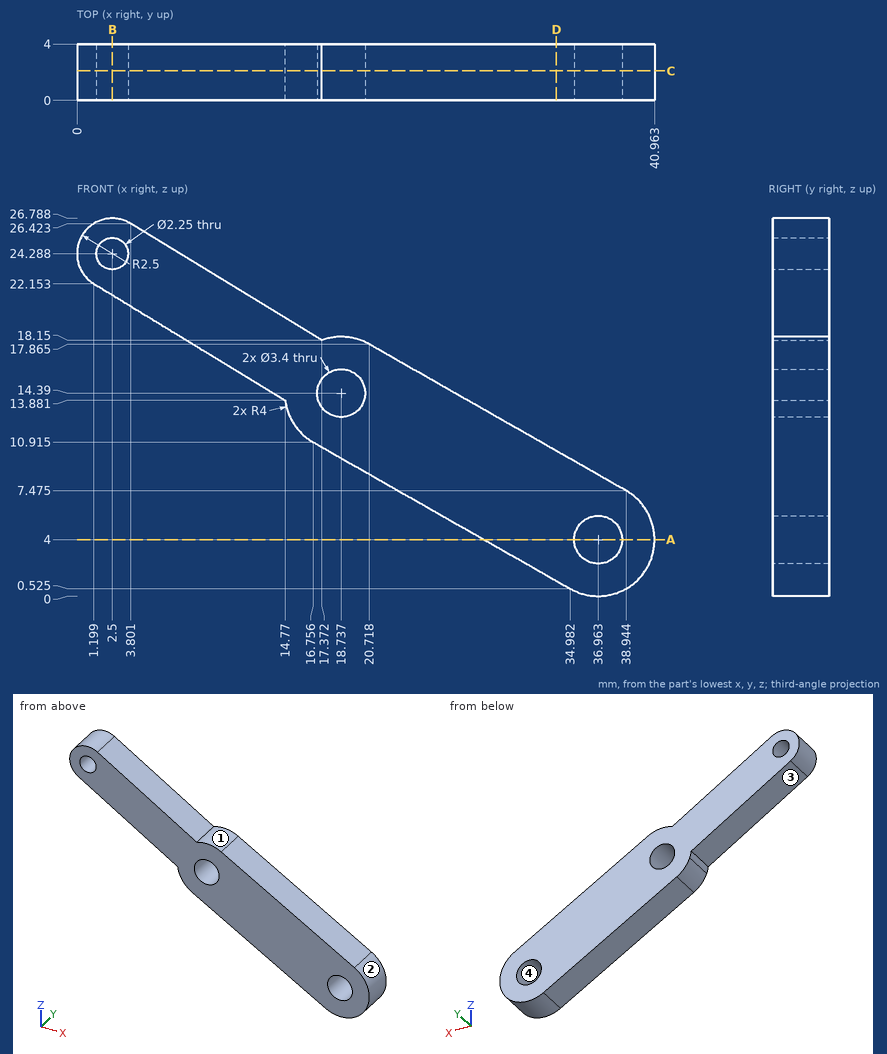
Here's the drawing with two shaded views (mm, measured from the low corner). I have some questions. Round coordinates to 2 decimals unless told otherwise and drop trailing zeros. Write each loop counter-clockwise with the first axis right and the second up, starting at its lowest first coordinate (ties: lowest second). Pieces come first, ordered by that corner, then holes. Notation, with made-up numbers: M 41,-18.5 L 46,-18.5 A23 cw 46,1.5 Z; hole C 56.5,-1.75 d4. An arc over 180 degrees is marked long. Use CSV: the item, a comma, the result in double quotes.
(1) Imagine slicing it at D-D (x = 34). Write out the boundary of the cut face in (y, z) (1 decimal).
Check values:
outline,"M 0,1.1 L 4,1.1 L 4,10.3 L 0,10.3 Z"
(2) We'd pull the mould along X, two halves only. Please class the marked faces 1, 2, 3 and 4: +X half, -X half, draft (parallel to the pull), parting line (faces both ways), or undercut.
Check values:
face 1,"undercut"
face 2,"parting line"
face 3,"-X half"
face 4,"undercut"
(3) Imagine slicing it at C-C (y = 2.1). Count the separate pieces of the cut face and the enclosed holes in it, plus the area to 3 significant figures.
Check values:
separate pieces,"1"
enclosed holes,"3"
area,"282 mm^2"
(4) I need wall thicknesses on line 1 along X through (y, z) = (1.95, 14) (1 decimal); line 2 along X through (y, z) = (2.15, 24.75) (1 decimal); line 3 along X through (y, z) = (2, 16.5) (1 decimal). Which ranges of each line are inside material? Lowest first, please.
Check values:
line 1,"14.6 to 17.1, 20.4 to 27.5"
line 2,"0 to 1.5, 3.5 to 6.5"
line 3,"10.5 to 23.1"
(5) Imagine slicing it at B-B (x = 2.5). Write out the boundary of the cut face in (y, z), plus the area to 3 significant figures.
Check values:
outline,"M 0,21.36 L 4,21.36 L 4,23.16 L 0,23.16 Z; M 0,25.41 L 4,25.41 L 4,26.79 L 0,26.79 Z"
area,"12.7 mm^2"
(6) Imagine slicing it at A-A (z = 4). Write out the boundary of the cut face in (x, y), plus the area to 3 significant figures.
Check values:
outline,"M 28.89,0 L 35.26,0 L 35.26,4 L 28.89,4 Z; M 38.66,0 L 40.96,0 L 40.96,4 L 38.66,4 Z"
area,"34.7 mm^2"
(7) I'm going to push flat-ended pins straight in: pin 1 (2 mm diameter, centred on y = 2.5, z = 17, fed in from +X); pin 2 (1.5 mm diameter, centred on y = 3, z = 13.5, fed in from +X); pin 3 (1.5 mm diameter, centred on x = 5.5, y = 3, fed in from +Z) (1 decimal). Where does each tip first touch, or does it pass through?
Check values:
pin 1,"x = 23.99"
pin 2,"x = 29.69"
pin 3,"z = 25.8"
